Here's how the part is built. I have some questions about the finished solid (model axes, mm). Give positions to 0.01 mm unless a question says otherwise; leave off trailing zeros. Loops run counter-clockwise (first coordinate to the right, second up) from the corner with the lowest first, then second, coordinate; pieces in that order, holes last. Notation, with made-up numbers: (30.25, 16.25) - (42.25, 16.25) arc R16 cw to (42.25, 43.25) - close; hole circle Ø7 at (-15.75, 19). An arc over 180 degrees is marked (long way). Put each result on its own line as item: value. Start each with the question number.
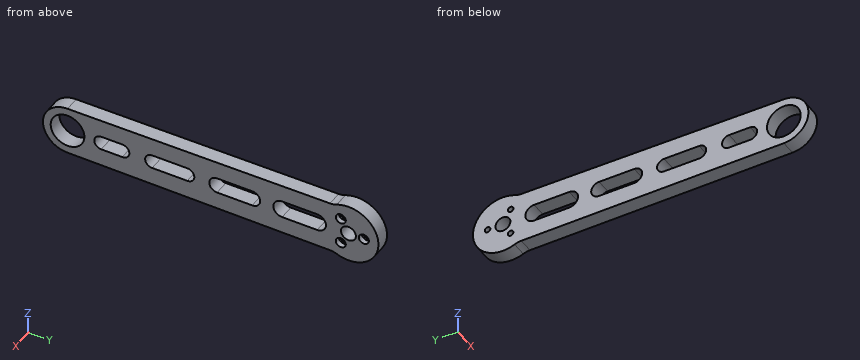
from build123d import *

# Parameters (mm, degrees)
SKETCH_3_R          = 9.6
EXTRUDE_1_DEPTH     = 8.5
SKETCH_4_R          = 4.25
SKETCH_4_R_2        = 1.6
CUT_EXTRUDE_1_DEPTH = 10
SKETCH_5_R          = 2.85
CUT_EXTRUDE_2_DEPTH = 3
CUT_EXTRUDE_3_DEPTH = 10
FILLET_1_R          = 10


with BuildPart() as part:
    # 草图3 → 凸台-拉伸1 (new body)
    with BuildSketch(Plane(origin=(0, 0, 0), x_dir=(0, 0, -1), z_dir=(1, 0, 0))):
        with BuildLine():
            Line((14, -160), (14.948368861, -8.260982254))
            ThreePointArc((14.948368861, -8.260982254), (0, 17.0791557), (-14.948368861, -8.260982254))
            Line((-14.948368861, -8.260982254), (-14, -160))
            ThreePointArc((-14, -160), (0, -174), (14, -160))
        make_face()
        with Locations((0, -160)):
            Circle(SKETCH_3_R, mode=Mode.SUBTRACT)
    extrude(amount=EXTRUDE_1_DEPTH)

    # 草图4 → 切除-拉伸1 (cut)
    with BuildSketch(Plane(origin=(8.5, 0, 0), x_dir=(0, 0, -1), z_dir=(1, 0, 0))):
        Circle(SKETCH_4_R)
        with Locations((0, 8.75)):
            Circle(SKETCH_4_R_2)
        with Locations((7.577722283, -4.375)):
            Circle(SKETCH_4_R_2)
        with Locations((-7.577722283, -4.375)):
            Circle(SKETCH_4_R_2)
    extrude(amount=-CUT_EXTRUDE_1_DEPTH, mode=Mode.SUBTRACT)

    # 草图5 → 切除-拉伸2 (cut)
    with BuildSketch(Plane(origin=(8.5, 0, 0), x_dir=(0, 0, -1), z_dir=(1, 0, 0))):
        with Locations((0, 8.75)):
            Circle(SKETCH_5_R)
        with Locations((7.577722283, -4.375)):
            Circle(SKETCH_5_R)
        with Locations((-7.577722283, -4.375)):
            Circle(SKETCH_5_R)
    extrude(amount=-CUT_EXTRUDE_2_DEPTH, mode=Mode.SUBTRACT)

    # 草图6 → 切除-拉伸3 (cut)
    with BuildSketch(Plane(origin=(8.5, 0, 0), x_dir=(0, 0, -1), z_dir=(1, 0, 0))):
        with BuildLine():
            Line((5, -17.788825977), (5, -37.788825977))
            ThreePointArc((5, -37.788825977), (0, -42.788825977), (-5, -37.788825977))
            Line((-5, -37.788825977), (-5, -17.788825977))
            ThreePointArc((-5, -17.788825977), (0, -12.788825977), (5, -17.788825977))
        make_face()
        with BuildLine():
            Line((4.5, -54.788825977), (4.5, -74.788825977))
            ThreePointArc((4.5, -74.788825977), (0, -79.288825977), (-4.5, -74.788825977))
            Line((-4.5, -74.788825977), (-4.5, -54.788825977))
            ThreePointArc((-4.5, -54.788825977), (0, -50.288825977), (4.5, -54.788825977))
        make_face()
        with BuildLine():
            Line((4, -91.788825977), (4, -111.788825977))
            ThreePointArc((4, -111.788825977), (0, -115.788825977), (-4, -111.788825977))
            Line((-4, -111.788825977), (-4, -91.788825977))
            ThreePointArc((-4, -91.788825977), (0, -87.788825977), (4, -91.788825977))
        make_face()
        with BuildLine():
            Line((4, -128.788825977), (4, -140.788825977))
            ThreePointArc((4, -140.788825977), (0, -144.788825977), (-4, -140.788825977))
            Line((-4, -140.788825977), (-4, -128.788825977))
            ThreePointArc((-4, -128.788825977), (0, -124.788825977), (4, -128.788825977))
        make_face()
    extrude(amount=-CUT_EXTRUDE_3_DEPTH, mode=Mode.SUBTRACT)

    # 圆角1
    fillet_1_edges = [part.edges().sort_by_distance(p)[0] for p in [
        (4.25, -8.260982254, 14.948368861),
        (4.25, -8.260982254, -14.948368861),
    ]]
    fillet(fillet_1_edges, radius=FILLET_1_R)


solid = part.part
1) I'm going to push flat-ended pins straight in: P1, Ø3, axis at x = 4.5, y = -46, coming from the -Z side; P2, Ø2.5, axis at x = 2.5, y = -61.5, coming from the +Z side; P3, Ø1, axis at y = -59, z = -2.5, coming from the +X side; P4, Ø4, axis at x = 1.5, y = -103, coming from the +Z side. Where does each tip first touch, or does it pass through?
2) Suppose I cut it at A-A on y = 8.75. Please give me the cut outline in (x, z), plus the area to 3 significant figures.
3) I need wall thicknesses on line 1 (Y direction, x = 5.75, z = 5.5); line 2 (Y direction, x = 5.75, z = 6); line 3 (Z direction, x = 7.5, y = -96.5). Which ranges of each line are inside material? Lowest first, please.
4) Suppose I cut it at B-B on x = 3. Give the number of separate pieces and of enclosed holes in the cut face, plus the area to 3 significant figures.
Ans:
1. P1: stops at z = -14.72
1. P2: stops at z = 14.62
1. P3: passes through
1. P4: stops at z = 14.37
2. outline: (0, -14.67) - (8.5, -14.67) - (8.5, -2.85) - (5.5, -2.85) - (5.5, -1.6) - (0, -1.6) - close; (0, 1.6) - (5.5, 1.6) - (5.5, 2.85) - (8.5, 2.85) - (8.5, 14.67) - (0, 14.67) - close
2. area: 215 mm²
3. line 1: y = -172.87 to -167.87, -152.13 to -6.33, -2.42 to 16.17
3. line 2: y = -172.65 to -167.49, -152.51 to -6.75, -2 to 15.99
3. line 3: z = -14.4 to -4, 4 to 14.4
4. separate pieces: 1
4. enclosed holes: 9
4. area: 4,180 mm²
